Could you check a few things on this model? Use its own coordinates, in mm. Give positions to 0.01 mm unless a question says otherwise; leave off trailing zeros. Loops run counter-clockwise (first coordinate to the right, second up) from the corner with the lowest first, then second, coordinate; pieces in that order, holes last. Notation, with made-up numbers: M 86.25,60.25 L 107.25,60.25 A29 ccw 107.25,85.25 Z; hole C 32,-28.75 d3. An arc over 180 degrees is marked long. Use a Markdown table: item, result. Add a question column.
1) Suppose I cut it at D-D on y = 162.5. List the corners of the cut face in (x, z) for me.
2) Will these pins go through, and if not, where does the flat tip stop? pin 1 Ø0.9 at (y, z) = (27, 2) entering from -X; pin 2 Ø1.5 at (x, z) = (-184.5, 1.5) entering from -Y; pin 3 Ø1.5 at (y, z) = (20, 1) entering from +X.
3) Suppose I cut it at C-C on z = 1.9. List the corners of the cut face in (x, y) for me.
4) If I drill on line 1 along Y through (x, z) = (-53, 2.15); line 2 along Y through (x, z) = (-27, 0.45); line 3 along Y through (x, z) = (-177, 0.3), over which ranges is the centre line in solid material (lowest first)? Write a range as [from, to].
5) Suppose I cut it at B-B on x = -164.5. List the corners of the cut face in (y, z) for me, and give its area (3 significant figures).
6) Suppose I cut it at A-A on y = 74. List the corners of the cut face in (x, z) for me.
```python
from build123d import *

# Parameters (mm, degrees)
BASE_DEPTH              = 3
PROFIL_S_DEPTH          = 3
ESQUISSE3_W             = 180
ESQUISSE3_H             = 20
ESQUISSE3_W_2           = 20
ESQUISSE3_H_2           = 70
ENL_V_MAT_EXTRU_1_DEPTH = 3


with BuildPart() as part:
    # Esquisse1 → Base (new body)
    with BuildSketch(Plane.XY):
        Polygon((0, 0), (-200, 0), (-224.748737342, 24.748737342), (-224.748737342, 284.748737342), (-200, 309.497474683), (0, 309.497474683), (24.748737342, 284.748737342), (24.748737342, 24.748737342), align=None)
    extrude(amount=BASE_DEPTH)

    # Esquisse2 → profilés (cut)
    with BuildSketch(Plane.XY.offset(3)):
        Polygon((-45, 13), (-155, 13), (-155, 33.5), (-224.748737342, 33.5), (-224.748737342, 0), (24.748737342, 0), (24.748737342, 33.5), (-45, 33.5), align=None)
        Polygon((24.748737342, 309.497474683), (24.748737342, 275.997474683), (-45, 275.997474683), (-45, 296.497474683), (-155, 296.497474683), (-155, 275.997474683), (-224.748737342, 275.997474683), (-224.748737342, 309.497474683), align=None)
    extrude(amount=-PROFIL_S_DEPTH, mode=Mode.SUBTRACT)

    # Esquisse3 → Enlèv. mat.-Extru.1 (cut)
    with BuildSketch(Plane.XY.offset(3)):
        with Locations((-100, 234.497474683)):
            Rectangle(ESQUISSE3_W, ESQUISSE3_H)
        with Locations((-100, 75)):
            Rectangle(ESQUISSE3_W, ESQUISSE3_H)
        with Locations((-184.748737342, 154.748737342)):
            Rectangle(ESQUISSE3_W_2, ESQUISSE3_H_2)
    extrude(amount=-ENL_V_MAT_EXTRU_1_DEPTH, mode=Mode.SUBTRACT)


solid = part.part
```
Answer block:
| question | item | result |
|---|---|---|
| 1 | outline | M -224.75,0 L -194.75,0 L -194.75,3 L -224.75,3 Z; M -174.75,0 L 24.75,0 L 24.75,3 L -174.75,3 Z |
| 2 | pin 1 | stops at x = -155 |
| 2 | pin 2 | stops at y = 33.5 |
| 2 | pin 3 | stops at x = -45 |
| 3 | outline | M -224.75,33.5 L -155,33.5 L -155,13 L -45,13 L -45,33.5 L 24.75,33.5 L 24.75,276 L -45,276 L -45,296.5 L -155,296.5 L -155,276 L -224.75,276 Z; hole M -194.75,119.75 L -174.75,119.75 L -174.75,189.75 L -194.75,189.75 Z; hole M -190,65 L -10,65 L -10,85 L -190,85 Z; hole M -190,224.5 L -10,224.5 L -10,244.5 L -190,244.5 Z |
| 4 | line 1 | y = [13, 65], [85, 224.5], [244.5, 296.5] |
| 4 | line 2 | y = [33.5, 65], [85, 224.5], [244.5, 276] |
| 4 | line 3 | y = [33.5, 65], [85, 119.75], [189.75, 224.5], [244.5, 276] |
| 5 | outline | M 33.5,0 L 65,0 L 65,3 L 33.5,3 Z; M 85,0 L 224.5,0 L 224.5,3 L 85,3 Z; M 244.5,0 L 276,0 L 276,3 L 244.5,3 Z |
| 5 | area | 607 mm^2 |
| 6 | outline | M -224.75,0 L -190,0 L -190,3 L -224.75,3 Z; M -10,0 L 24.75,0 L 24.75,3 L -10,3 Z |
